For this review, take the finished solid that the model builds, in its own axes (mm). A direction names the side the tool comes from. Coordinates: 2 decimals unless noted, no trailing zeros. Loops run counter-clockwise (first coordinate to the right, second up) from the corner with the lowest first, then second, coordinate; pieces in that order, holes last. Notation, with made-up numbers: M -38.5,-10.5 L -17.5,-10.5 A21 cw -17.5,2.5 Z; hole C -35,75.25 d3. An arc over 180 degrees is marked long. Answer as a JSON object with one key per item and string values. Group by question number.
Item 1: Tool access review of faces 1 (the face through (-9.781, 14.664, 0.74)), 2 (the face through (-11.821, 4, 1)), 3 (the face through (0, 16.566, 6)), 4 (the face through (0, 0.791, 8)), 5 (the face through (-7.821, 9, 8)): name each direction out of +Z, -Z, +X, -X, +Y, -Y from which nothing blocks a thin tool from reaching the whole face with its end or side.
Item 2: Add section A-A (y = 4.75). State the section outline as (x, z) points, then the cut area to 3 significant figures.
Item 3: Insertion check: pin 1 (2.5 mm diameter, centred on x = 11.38, y = 14.19, fed in from +Z); pin 2 (4.5 mm diameter, centred on x = -9.3, y = -4.74, fed in from -Z); pin 3 (1.1 mm diameter, centred on x = -10.77, y = 16.02, fed in from +Z); pin 4 (3 mm diameter, centred on x = -1.5, z = 9, fed in from +Y). Each pin has a flat end and moves straight along its axis. Give the tip position at first contact, or say it passes through.
Item 4: Add section D-D (z = 6.25). State the section outline as (x, y) points.
Item 5: Mouldability with a two-part tool opening along Y and no side actions: class faces 6 (the face through (15, 12.191, 1)), 7 (the face through (16.529, 14, 1)), 8 (the face through (10.7, 13.6, 2.2)) as +Y half, -Y half, draft (parallel to the pull), parting line (faces both ways), or undercut.
Item 6: Add section B-B (z = 2.25). State the section outline as (x, y) points (3 decimals), then the cut area to 3 significant figures.
Item 7: Add section C-C (x = -0.75). State the section outline as (y, z) points, then the cut area to 3 significant figures.
Item 8: Wall thickness on L1, parallel to X at y = 3.25, z = 5.75; L2, parallel to Y at x = -6.25, z = 7; L3, parallel to Y at x = 5.5, z = 2.75: over which ranges is each line inside the solid? List them lowest first. Write a range as from..to.
Autodesk Inventor part; units mm, degrees
ref_plane "Arbeitsebene1" through (-9.7716, -9.2098, 6) normal (0, 0, 1) x (1, 0, 0)
ref_plane "YZ Plane" through (0, 0, 0) normal (1, 0, 0) x (0, 1, 0)
ref_plane "XZ Plane" through (0, 0, 0) normal (0, 1, 0) x (-1, 0, 0)
sketch "Skizze1" plane through (0, 0, 0) normal (0, 0, 1) x (1, 0, 0)
  line L0 (14.1792, -17.284) -> (14.1792, 17.716)
  line L1 (14.1792, 17.716) -> (-11.8208, 17.716)
  line L2 (-11.8208, 17.716) -> (-11.8208, -17.284)
  line L3 (-11.8208, -17.284) -> (14.1792, -17.284)
  line L4 (14.1792, -17.284) -> (-11.8208, 17.716) construction
  line L5 (14.1792, 17.716) -> (-11.8208, -17.284) construction
  line L6 (3.4292, 10.341) -> (-6.0708, 10.341) construction
  line L7 (3.4292, 3.091) -> (3.4292, 10.341) construction
  line L8 (-6.0708, 3.091) -> (3.4292, 3.091) construction
  line L9 (-6.0708, 10.341) -> (-6.0708, 3.091) construction
  line L10 (3.4292, 10.341) -> (-6.0708, 3.091) construction
  line L11 (3.4292, 3.091) -> (-6.0708, 10.341) construction
  point P0 (0, 0)
  point P1 (1.1792, 0.216)
  point P2 (1.1792, 0.216)
  point P3 (-1.3208, 6.716)
  point P4 (-1.3208, 6.716)
  point P5 (1.1792, 0.216)
  point P6 (-1.3208, 6.716)
  dimension "d0" = 26
  dimension "d1" = 35
  dimension "d2" = 11
  dimension "d3" = 2.5
sketch "Skizze2" plane through (0, 0, 0) normal (0, 0, 1) x (1, 0, 0)
  line L0 (-3.4208, 1.091) -> (-7.8208, 1.091)
  line L1 (-7.8208, 1.091) -> (-7.8208, 12.341)
  line L2 (-7.8208, 12.341) -> (-3.4208, 12.341)
  line L3 (5.1792, 1.091) -> (0.7792, 1.091)
  line L4 (5.1792, 12.341) -> (5.1792, 1.091)
  line L5 (0.7792, 12.341) -> (5.1792, 12.341)
  circle A0 centre (-9.3002, -4.7384) radius 1.575 construction
  circle A1 centre (11.3792, 14.191) radius 1.575 construction
  circle A2 centre (-9.3002, -4.7384) radius 0.7 construction
  circle A3 centre (-10.7708, 16.016) radius 0.7 construction
  circle A4 centre (11.3792, 14.191) radius 0.7 construction
  line L6 (-3.4208, 12.341) -> (-3.4208, 13.366)
  line L7 (-3.4208, 13.366) -> (0.7792, 13.366)
  line L8 (0.7792, 0.066) -> (-3.4208, 0.066)
  line L9 (-3.4208, 0.066) -> (-3.4208, 1.091)
  line L10 (0.7792, 1.091) -> (0.7792, 0.066)
  line L11 (0.7792, 13.366) -> (0.7792, 12.341)
  line L12 (-12.2708, -9.259) -> (-12.2708, 10.741) construction
  line L13 (14.5292, 16.566) -> (-9.295, 16.566) construction
  arc A5 (16.5292, 14.566) -> (14.5292, 16.566) centre (14.5292, 14.566) ccw
  line L14 (16.5292, 14.566) -> (16.5292, 13.191)
  arc A6 (15.5292, 12.191) -> (16.5292, 13.191) centre (15.5292, 13.191) ccw
  line L15 (15.5292, 12.191) -> (14.4292, 12.191)
  arc A7 (14.4292, 12.191) -> (12.4292, 10.191) centre (14.4292, 10.191) ccw
  line L16 (12.4292, 10.191) -> (12.4292, -3.209)
  line L17 (-3.5708, -3.209) -> (12.4292, -3.209)
  line L18 (-8.1002, -7.7384) -> (-3.5708, -3.209)
  arc A8 (-10.7708, 17.591) -> (-9.295, 16.566) centre (-10.7708, 16.016) ccw construction
  line L19 (-8.1002, -8.7384) -> (-8.1002, -7.7384) construction
  circle A9 centre (-9.3002, -8.7384) radius 0.75 construction
  circle A10 centre (-9.3002, -8.7384) radius 1.2 construction
  line L20 (-10.8208, -7.909) -> (-11.8208, -6.909) construction
  line L21 (-11.8208, -6.909) -> (-11.8208, 14.7109)
  line L22 (-11.8208, -6.909) -> (-10.4976, -8.2322)
  arc A11 (-8.1002, -8.2384) -> (-8.2864, -7.9246) centre (-9.3002, -8.7384) ccw construction
  line L23 (-8.1002, -8.2384) -> (-8.1002, -7.7384) construction
  circle A12 centre (-9.3002, -4.7384) radius 1.675
  circle A13 centre (11.3792, 14.191) radius 1.675
  line L24 (14.5292, 16.566) -> (-9.1887, 16.566)
  arc A14 (-11.8208, 14.7109) -> (-9.1887, 16.566) centre (-10.7708, 16.016) ccw
  circle A15 centre (14.3792, 14.191) radius 0.75 construction
  circle A16 centre (14.3792, 14.191) radius 0.85
  line L25 (-8.1002, -7.7384) -> (-8.2864, -7.9246) construction
  arc A17 (-8.2864, -7.9246) -> (-10.4976, -8.2322) centre (-9.3002, -8.7384) ccw construction
  line L26 (-11.8208, -6.909) -> (-7.2708, -6.909)
  point P0 (0, 0)
  dimension "d4" = 0.1
  dimension "d5" = 0.1
  dimension "d6" = 0.1
  dimension "d7" = 0.1
  dimension "d10" = 0.1
extrude "Extrusion1" add sketch "Skizze2" along normal blind 1.5 contours L0 L1 L2 L6 L7 L11 L5 L4 L3 L10 L8 L9 | L14 A6 L15 A7 L16 L17 L18 L26 L21 A14 L24 A5
sketch "Skizze3" plane through (0, 0, 1.5) normal (0, 0, 1) x (1, 0, 0)
  circle A0 centre (11.3792, 14.191) radius 1.675 construction
  circle A1 centre (-9.3002, -4.7384) radius 1.675 construction
  circle A2 centre (14.3792, 14.191) radius 0.85
  arc A3 (16.5292, 14.566) -> (14.5292, 16.566) centre (14.5292, 14.566) ccw
  line L0 (14.5292, 16.566) -> (-9.1887, 16.566)
  arc A4 (-11.8208, 14.7109) -> (-9.1887, 16.566) centre (-10.7708, 16.016) ccw construction
  line L1 (-11.8208, 14.7109) -> (-11.8208, -6.909)
  line L2 (-7.2708, -6.909) -> (-3.5708, -3.209)
  line L3 (-3.5708, -3.209) -> (12.4292, -3.209)
  line L4 (12.4292, -3.209) -> (12.4292, 10.191)
  arc A5 (14.4292, 12.191) -> (12.4292, 10.191) centre (14.4292, 10.191) ccw
  line L5 (14.4292, 12.191) -> (15.5292, 12.191)
  arc A6 (15.5292, 12.191) -> (16.5292, 13.191) centre (15.5292, 13.191) ccw
  line L6 (16.5292, 13.191) -> (16.5292, 14.566)
  circle A7 centre (11.3792, 14.191) radius 0.7 construction
  circle A8 centre (-9.3002, -4.7384) radius 0.7 construction
  circle A9 centre (-9.3002, -8.7384) radius 0.75 construction
  circle A10 centre (-9.3002, -8.7384) radius 0.85
  line L7 (-7.2708, -6.909) -> (-3.5708, -3.209)
  arc A11 (-10.4976, -8.2322) -> (-8.2864, -7.9246) centre (-9.3002, -8.7384) ccw
  arc A12 (-9.1887, 16.566) -> (-11.8208, 14.7109) centre (-10.7708, 16.016) ccw
  circle A13 centre (-10.7708, 16.016) radius 0.7 construction
  circle A14 centre (-10.7708, 16.016) radius 0.9
  circle A15 centre (11.3792, 14.191) radius 0.9
  circle A16 centre (-9.3002, -4.7384) radius 0.9
  line L8 (-11.8208, -6.909) -> (-7.2708, -6.909)
  point P0 (0, 0)
  dimension "d11" = 0.1
  dimension "d13" = 1.8
  dimension "d14" = 1.8
  dimension "d15" = 1.8
ref_plane "Arbeitsebene1" through (-9.7716, -9.2098, 6) normal (0, 0, 1) x (1, 0, 0)
extrude "Extrusion2" add sketch "Skizze3" along normal blind 1.5 contours L6 A6 L5 A5 L4 L3 L2 L8 L1 A12 L0 A3
sketch "Skizze4" plane through (-9.1887, 16.566, 3) normal (0, 0, 1) x (1, 0, 0)
  circle A0 centre (-0.1115, -21.3043) radius 0.7 construction
  circle A1 centre (-1.5821, -0.55) radius 0.7 construction
  circle A2 centre (20.5679, -2.375) radius 0.7 construction
  point P0 (9.1887, -16.566)
sketch "Sketch8" plane through (0, 0, 3) normal (0, 0, 1) x (1, 0, 0)
  circle A0 centre (-10.7708, 16.016) radius 0.9
  circle A1 centre (14.3792, 14.191) radius 0.85
  arc A2 (16.5292, 14.566) -> (14.5292, 16.566) centre (14.5292, 14.566) ccw
  line L0 (14.5292, 16.566) -> (-9.1887, 16.566)
  arc A3 (-9.1887, 16.566) -> (-11.8208, 14.7109) centre (-10.7708, 16.016) ccw
  line L1 (-11.8208, 14.7109) -> (-11.8208, -6.909)
  line L2 (-11.8208, -6.909) -> (-7.2708, -6.909)
  line L3 (-3.5708, -3.209) -> (12.4292, -3.209)
  line L4 (12.4292, -3.209) -> (12.4292, 10.191)
  arc A4 (14.4292, 12.191) -> (12.4292, 10.191) centre (14.4292, 10.191) ccw
  line L5 (14.4292, 12.191) -> (15.5292, 12.191)
  arc A5 (15.5292, 12.191) -> (16.5292, 13.191) centre (15.5292, 13.191) ccw
  line L6 (16.5292, 13.191) -> (16.5292, 14.566)
  line L7 (-7.2708, -6.909) -> (-3.5708, -3.209)
  line L8 (-7.8208, 16.566) -> (8.4292, 16.566)
  line L9 (8.4292, 16.566) -> (8.4292, 0.791)
  line L10 (8.4292, 0.791) -> (-7.8208, 0.791)
  line L11 (-7.8208, 0.791) -> (-7.8208, 16.566)
  dimension "d37" = 4
  dimension "d38" = 4
  dimension "d39" = 4
  dimension "d40" = 0
extrude "Extrusion6" add sketch "Sketch8" along normal blind 10 contours L9 L10 L11 L0
properties part number "Raman2Go_Adapterplatte2_XY-TischChina"
From the geometry:
{
 "1": {"face 1": "-Z", "face 2": "+Z, -Z, -X, -Y", "face 3": "+Z, -Z, +X, +Y", "face 4": "+Z, +X, -X, -Y", "face 5": "+Z, -X, +Y, -Y"},
 "2": {"outline": "M -11.82,0 L 12.43,0 L 12.43,3 L 8.43,3 L 8.43,13 L -7.82,13 L -7.82,3 L -11.82,3 Z", "area": "235 mm²"},
 "3": {"pin 1": "stops at z = 3", "pin 2": "stops at z = 0", "pin 3": "passes through", "pin 4": "stops at y = 16.57"},
 "4": {"outline": "M -7.82,0.79 L 8.43,0.79 L 8.43,16.57 L -7.82,16.57 Z"},
 "5": {"face 6": "-Y half", "face 7": "draft", "face 8": "undercut"},
 "6": {"outline": "M -11.821,-6.909 L -7.271,-6.909 L -3.571,-3.209 L 12.429,-3.209 L 12.429,10.191 A2 cw 14.429,12.191 L 15.529,12.191 A1 ccw 16.529,13.191 L 16.529,14.566 A2 ccw 14.529,16.566 L -9.189,16.566 A1.675 ccw long -11.821,14.711 Z; hole C -10.771,16.016 d1.8; hole C -9.3,-4.738 d1.8; hole C 11.379,14.191 d1.8; hole C 14.379,14.191 d1.7", "area": "515 mm²"},
 "7": {"outline": "M -3.21,0 L 16.57,0 L 16.57,13 L 0.79,13 L 0.79,3 L -3.21,3 Z", "area": "217 mm²"},
 "8": {"L1": "x = -7.82..8.43", "L2": "y = 0.79..16.57", "L3": "y = -3.21..16.57"}
}
